```python
from build123d import *
from build123d.topology import SkipClean

# Parameters (mm, degrees)
BOSS_EXTRUDE1_DEPTH       = 12.7
CUT_EXTRUDE1_DEPTH        = 12.7
BOSS_EXTRUDE2_OUTLINE_R   = 75
BOSS_EXTRUDE2_OUTLINE_R_2 = 2.05
BOSS_EXTRUDE2_DEPTH       = 6
SKETCH3_4_R               = 80
SKETCH3_4_R_2             = 75
BOSS_EXTRUDE3_DEPTH       = 15
SKETCH4_R                 = 3.5
CUT_EXTRUDE2_DEPTH        = 4.2


with BuildPart() as part:
    # Sketch1 → Boss-Extrude1 (new body)
    with BuildSketch(Plane(origin=(0, 0, 0), x_dir=(1, 0, 0), z_dir=(0, 1, 0))):
        Polygon((-58.57612782, 0), (16.42387218, 0), (16.42387218, 5), (-37.711466165, 5), (-37.711466165, 10), (-58.57612782, 10), align=None)
    extrude(amount=BOSS_EXTRUDE1_DEPTH)

    # Sketch2 → Cut-Extrude1 (cut)
    with BuildSketch(Plane(origin=(0, 0, -10), x_dir=(-1, 0, 0), z_dir=(0, 0, -1))):
        with BuildLine():
            ThreePointArc((41.243796992, 6.35), (43.293796992, 4.3), (45.343796992, 6.35))
            Line((45.343796992, 6.35), (41.243796992, 6.35))
        make_face()
        with BuildLine():
            Line((41.243796992, 6.35), (45.343796992, 6.35))
            ThreePointArc((45.343796992, 6.35), (43.293796992, 8.4), (41.243796992, 6.35))
        make_face()
        with BuildLine():
            ThreePointArc((55.043796992, 6.35), (52.993796992, 8.4), (50.943796992, 6.35))
            Line((50.943796992, 6.35), (55.043796992, 6.35))
        make_face()
        with BuildLine():
            Line((55.043796992, 6.35), (50.943796992, 6.35))
            ThreePointArc((50.943796992, 6.35), (52.993796992, 4.3), (55.043796992, 6.35))
        make_face()
    extrude(amount=-CUT_EXTRUDE1_DEPTH, mode=Mode.SUBTRACT)

    # Boss-Extrude2: read off the stored shape, not the designer's step
    # Boss-Extrude2 outline → Boss-Extrude2 (add)
    with SkipClean():  # the faces are left unmerged after this step: merging them gives an invalid solid
        with BuildSketch(Plane.XY):
            with Locations((0, 6.35)):
                Circle(BOSS_EXTRUDE2_OUTLINE_R)
            with Locations((-52.993796992, 6.35)):
                Circle(BOSS_EXTRUDE2_OUTLINE_R_2, mode=Mode.SUBTRACT)
            with Locations((-43.293796992, 6.35)):
                Circle(BOSS_EXTRUDE2_OUTLINE_R_2, mode=Mode.SUBTRACT)
        extrude(amount=BOSS_EXTRUDE2_DEPTH)

    # Sketch3_4 → Boss-Extrude3 (add)
    with SkipClean():  # the faces are left unmerged after this step: merging them gives an invalid solid
        with BuildSketch(Plane.XY):
            with Locations((0, 6.35)):
                Circle(SKETCH3_4_R)
            with Locations((0, 6.35)):
                Circle(SKETCH3_4_R_2, mode=Mode.SUBTRACT)
        extrude(amount=BOSS_EXTRUDE3_DEPTH)
    add(part.part.scale(1), mode=Mode.REPLACE)  # the faces are merged on a copy

    # Sketch4 → Cut-Extrude2 (cut)
    with SkipClean():  # the faces are left unmerged after this step: merging them gives an invalid solid
        with BuildSketch(Plane.XY.offset(6)):
            with Locations((-52.993796992, 6.35)):
                Circle(SKETCH4_R)
            with Locations((-43.293796992, 6.35)):
                Circle(SKETCH4_R)
        extrude(amount=-CUT_EXTRUDE2_DEPTH, mode=Mode.SUBTRACT)


solid = part.part
```
Geometry check sheet. Reference: the model listing, model coordinates, mm. A direction names the side the tool comes from. Coordinates: 2 decimals unless noted, no trailing zeros. Write each loop counter-clockwise with the first axis right and the second up, starting at its lowest first coordinate (ties: lowest second). Pieces come first, ordered by that corner, then holes. Notation, with made-up numbers: M -22.75,42 L 7.25,42 A36 ccw 7.25,79 Z; hole C -19.5,39.5 d1. An arc over 180 degrees is marked long. Use one line per item in the form item = value. Start each with the question number.
1) Section check D-D on y = 69. Enter the section's corners in (x, z), and give its area (3 significant figures).
2) Set-up check for faces 4 (the flat face through (-30, 12.7, -4)), 5 (the cylindrical face through (-9.764, 80.712, 10.437)), 6 (the flat face through (-58.576, 6, -5)): record each of +Z, -Z, +X, -X, +Y, -Y from which the full face is reachable in a straight line by a thin tool's end or side.
3) Thickness scan on probe 1 along Z at (x, y) = (-61, -26); probe 2 along Z at (x, y) = (69.5, -31); probe 3 along Y at (x, z) = (-48, 11.75). Record the ranges inside material, lowest first. Write a range as from..to.
4) Release check for a two-part mould opening along X. For faces 1 (the cylindrical face through (-40.06, 5.01, 3.93)), 2 (the flat face through (-10, 6, -5)), 3 (the cylindrical face through (76.3, 30.4, 7.4)) record: pulls with the +X half, pulls with the -X half, needs draft (parallel to the pull), parting line crosses it, or undercut.
5) Section check C-C on z = -8. Enter the section's corners in (x, y), and give its area (3 significant figures).
6) Section check B-B on x = 0. Enter the section's corners in (y, z), and give its area (3 significant figures).
7) Go/stop test with flat-tipped pins: pin 1 Ø4 at (y, z) = (-48, 2) entering from +X; pin 2 Ø9 at (x, y) = (-52.99, 6.35) entering from +Z; pin 3 Ø3 at (x, z) = (-6, -4) entering from -Y; pin 4 Ø3.5 at (x, y) = (-52.99, 6.35) entering from -Z. Record where each tip stops, or that it passes through.
8) Section check A-A on y = 6.35. State how many separate pieces and enclosed holes the cut face has, and give its area (3 significant figures).
Responses:
q1.outline = M -49.75,0 L 49.75,0 L 49.75,15 L 41.23,15 L 41.23,6 L -41.23,6 L -41.23,15 L -49.75,15 Z
q1.area = 750 mm2
q2.face_4 = -Z, +X, -X, +Y
q2.face_5 = +Z
q2.face_6 = -Z, -X, +Y, -Y
q3.probe_1 = 0..6
q3.probe_2 = 0..15
q3.probe_3 = -57.65..-51.28, 63.98..70.35
q4.face_1 = undercut
q4.face_2 = needs draft
q4.face_3 = parting line crosses it
q5.outline = M -58.58,0 L -37.71,0 L -37.71,12.7 L -58.58,12.7 Z; hole C -52.99,6.35 d4.1; hole C -43.29,6.35 d4.1
q5.area = 239 mm2
q6.outline = M -73.65,0 L 0,0 L 0,-5 L 12.7,-5 L 12.7,0 L 86.35,0 L 86.35,15 L 81.35,15 L 81.35,6 L -68.65,6 L -68.65,15 L -73.65,15 Z
q6.area = 1,110 mm2
q7.pin_1 = 60.49
q7.pin_2 = 6
q7.pin_3 = 0
q7.pin_4 = through
q8.separate_pieces = 3
q8.enclosed_holes = 0
q8.area = 1,370 mm2
